Solid Edge part; units mm, degrees
sketch "Sketch1" plane through (0, 0, 0) normal (0, 0, 1) x (1, 0, 0)
  line L0 (-23, -6) -> (23, -6)
  arc A0 (23, 6) -> (23, -6) centre (23, 0) cw
  line L1 (23, 6) -> (-23, 6)
  arc A1 (-23, 6) -> (-23, -6) centre (-23, 0) ccw
  arc A2 (-28.8095, 1.5) -> (-28.8095, -1.5) centre (-23, 0) ccw
  line L2 (-28.8095, -1.5) -> (-25, -1.5)
  line L3 (-25, -1.5) -> (-25, 1.5)
  line L4 (-25, 1.5) -> (-28.8095, 1.5)
extrude "Protrusion1" add sketch "Sketch1" against normal blind 2
fillet "Round_1" radius 2 4 edges at (0, -6, 0) (29, 0, 0) (0, 6, 0) (-29, 0, 0)
sketch "Sketch2" plane through (0, 0, 0) normal (0, 0, 1) x (1, 0, 0)
  line L0 (-28.8095, -1.5) -> (-25, -1.5)
  line L1 (-25, -1.5) -> (-25, 1.5)
  line L2 (-25, 1.5) -> (-28.8095, 1.5)
  arc A0 (-28.8095, 1.5) -> (-28.8095, -1.5) centre (-23, 0) ccw
extrude "ExtrudedCutout_1" cut sketch "Sketch2" against normal blind 2
sketch "Sketch3" plane through (0.0953, 0, -2) normal (0, 0, -1) x (-1, 0, 0)
  line L0 (-19.9047, -1.5) -> (25.0953, -1.5)
  line L1 (25.0953, -1.5) -> (25.0953, 1.5)
  line L2 (25.0953, 1.5) -> (-19.9047, 1.5)
  line L3 (-19.9047, 1.5) -> (-19.9047, -1.5)
extrude "ExtrudedCutout_2" cut sketch "Sketch3" against normal blind 1.25
sketch "Sketch4" plane through (0.0953, 0, -2) normal (0, 0, -1) x (-1, 0, 0)
  circle A0 centre (23.0953, -3) radius 1
extrude "ExtrudedCutout_3" cut sketch "Sketch4" against normal blind 1.75
sketch "Sketch5" plane through (0.0953, 0, -2) normal (0, 0, -1) x (-1, 0, 0)
  circle A0 centre (23.0953, 3) radius 1
extrude "ExtrudedCutout_4" cut sketch "Sketch5" against normal blind 1.75
sketch "Sketch6" plane through (0.0953, 0, -2) normal (0, 0, -1) x (-1, 0, 0)
  circle A0 centre (-22.9047, -3) radius 1
extrude "ExtrudedCutout_6" cut sketch "Sketch6" against normal blind 1.75
sketch "Sketch7" plane through (0.0953, 0, -2) normal (0, 0, -1) x (-1, 0, 0)
  circle A0 centre (-22.9047, 3) radius 1
extrude "ExtrudedCutout_7" cut sketch "Sketch7" against normal blind 1.75
sketch "Sketch8" plane through (0.0953, 0, -2) normal (0, 0, -1) x (-1, 0, 0)
  circle A0 centre (-25.9047, 0) radius 1.5
extrude "ExtrudedCutout_8" cut sketch "Sketch8" against normal blind 1
Source: CAD feature listing. Evaluate the final solid. Frame: model axes, mm. A direction names the side the tool comes from. Give positions to 0.01 mm unless a question says otherwise; leave off trailing zeros. Order: outer loops, then holes, each group sorted by start corner. A loop starts at its lowest first (then second) coordinate and runs counter-clockwise, first axis right, second up. Notation, with made-up numbers: (78, -38) -> (92, -38) arc R13 ccw to (92, -17) -> close; hole circle Ø3 at (-25, 76). An arc over 180 degrees is marked (long way). Write item = value, one per line.
Q1. Pin query (flat end, axial travel): pin 1 (1.5 mm diameter, centred on x = 26.5, y = 0, fed in from -Z); pin 2 (0.6 mm diameter, centred on x = 4, z = -1.5, fed in from -Y); pin 3 (0.6 mm diameter, centred on x = -26, z = -1.5, fed in from +Y). Return the tip coordinate at first contact, or that it passes through.
Data:
pin_1 = -1
pin_2 = -5.99
pin_3 = 5.3
Q2. Cut plane C-C, the plane z = -1.4. Output: boundary loops of the cut face in (x, y), and give its area (3 significant figures).
Data:
outline = (-28.71, -1.5) arc R5.91 ccw to (-23, -5.91) -> (23, -5.91) arc R5.91 ccw to (23, 5.91) -> (-23, 5.91) arc R5.91 ccw to (-28.71, 1.5) -> (-25, 1.5) -> (20, 1.5) -> (20, -1.5) -> (-25, -1.5) -> close; hole circle Ø2 at (-23, -3); hole circle Ø2 at (-23, 3); hole circle Ø2 at (23, -3); hole circle Ø2 at (23, 3); hole circle Ø3 at (26, 0)
area = 487 mm^2
Q3. Pull-direction query (Y, two-part tool) for faces 4 (the face through (0, 3, -2)), 5 (the face through (-22, -3, -1)), 6 (the face through (-0.32, -5.43, -0.6)); classes: released by +Y, released by -Y, zero draft, split by the parting line, or undercut.
Data:
face_4 = zero draft
face_5 = undercut
face_6 = released by -Y
Q4. Material intervals for line 1 (Y direction, x = -23, z = -0.8); line 2 (Y direction, x = 23, z = -1.15); line 3 (Y direction, x = 23, z = -1.3), sorted ascending. Write a range as from..to.
Data:
line_1 = -5.6..-4, -2..-1.5, 1.5..2, 4..5.6
line_2 = -5.81..-4, -2..2, 4..5.81
line_3 = -5.87..-4, -2..2, 4..5.87
Q5. Cut plane B-B, the plane x = 10. Output: boundary loops of the cut face in (y, z), and give its area (3 significant figures).
Data:
outline = (-6, -2) -> (-1.5, -2) -> (-1.5, -0.75) -> (1.5, -0.75) -> (1.5, -2) -> (6, -2) arc R2 ccw to (4, 0) -> (-4, 0) arc R2 ccw to start
area = 18.5 mm^2
Q6. Set-up query: faces 1 (the face through (0, 0, 0)), 2 (the face through (20, 0, -1)), 3 (the face through (-22.263, 3.676, -1.137)). Return all of +Z, -Z, +X, -X, +Y, -Y with unobstructed straight access to the full face (end or side cutting, diameter ignored); none if empty.
Data:
face_1 = +Z, +X, -X, +Y, -Y
face_2 = -Z, -X
face_3 = -Z
Q7. Cut plane A-A, the plane y = 0. Output: boundary loops of the cut face in (x, z), and give its area (3 significant figures).
Data:
outline = (-25, -0.75) -> (20, -0.75) -> (20, -2) -> (24.5, -2) -> (24.5, -1) -> (27.5, -1) -> (27.5, -2) -> (29, -2) arc R2 ccw to (27, 0) -> (-25, 0) -> close
area = 47.9 mm^2
